Here's the drawing with two shaded views (mm, measured from the low corner). I have some questions. A direction names the side the tool comes from. Give positions to 0.01 mm unless a question says otherwise; leave off trailing zeros. Loops run counter-clockwise (first coordinate to the right, second up) from the corner with the lowest first, then second, coordinate; pieces in that order, holes last. Notation, with made-up numbers: (3.5, 10.5) -> (17.5, 10.5) arc R30 ccw to (17.5, 43.5) -> close; hole circle Ø8 at (5.5, -9.5). An arc over 180 degrees is marked (long way). Answer in a Markdown table with one row per item. Add a question column.
Item 1: If we section it at B-B (y = 17.75): Write out the boundary of the cut face in (x, z), then the cut area to 3 significant figures.
Item 2: If we section it at C-C (y = 13.25): Write out the boundary of the cut face in (x, z).
Item 3: For P1, Ø3, axis at x = 17, z = 13.5, coming from the -Y side; P2, Ø3, axis at x = 19, y = 23.5, coming from the +Z side; P3, Ø2, axis at x = 21.5, z = 16, coming from the +Y side, each with a flat end and sliding along its axis, tell me the tip position at first contact or that it passes through.
Item 4: If we section it at A-A (x = 4.5): Write out the boundary of the cut face in (y, z), then the cut area to 3 significant figures.
Item 5: If I drill on line 1 (Z direction, x = 15.5, y = 24.25); line 2 (Y direction, x = 30, z = 29); line 3 (Y direction, x = 4, z = 16), over which ranges is the centre line in solid material (lowest first)?
Item 6: Which directions (+Z, -Z, +X, -X, +Y, -Y) give clear straight access to the entire face, cutting with the end or side of a thin tool? Please do the marked faces 1 and 2.
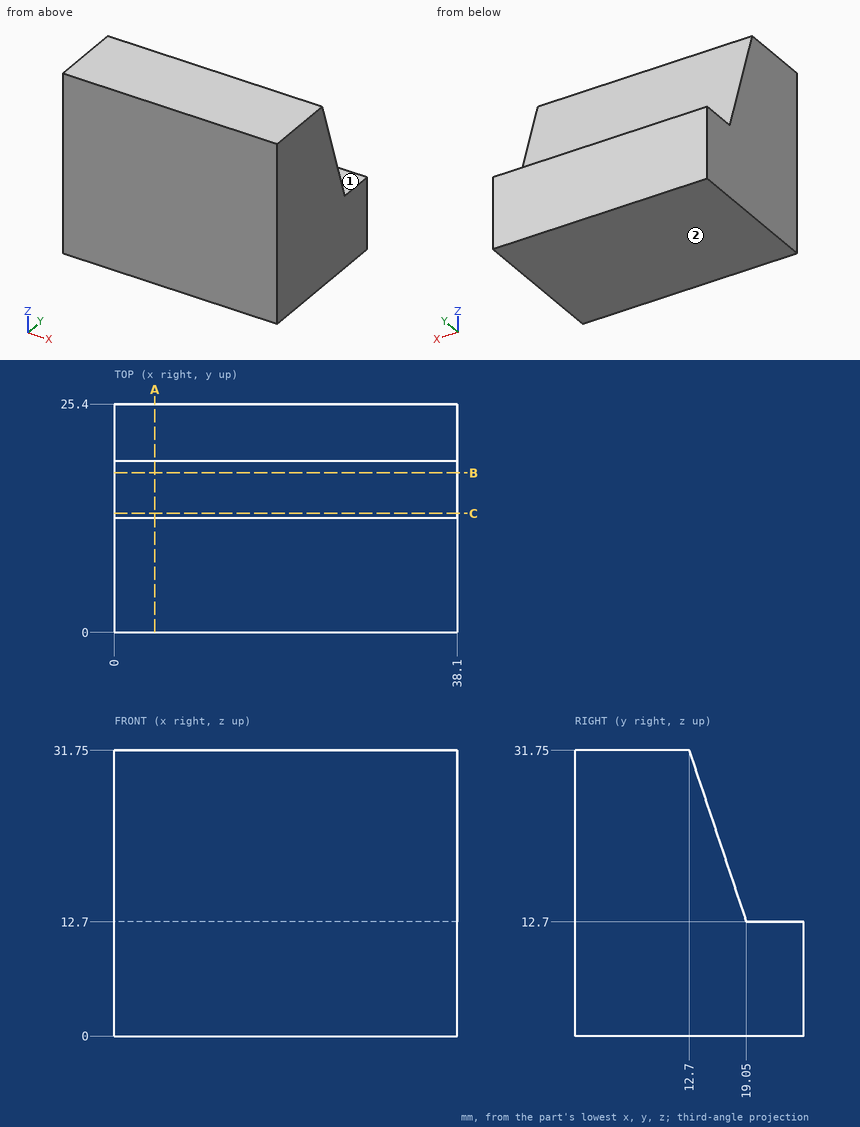
Recorded:
| question | item | result |
|---|---|---|
| 1 | outline | (0, 0) -> (38.1, 0) -> (38.1, 16.6) -> (0, 16.6) -> close |
| 1 | area | 632 mm^2 |
| 2 | outline | (0, 0) -> (38.1, 0) -> (38.1, 30.1) -> (0, 30.1) -> close |
| 3 | P1 | stops at y = 0 |
| 3 | P2 | stops at z = 12.7 |
| 3 | P3 | stops at y = 18.28 |
| 4 | outline | (0, 0) -> (25.4, 0) -> (25.4, 12.7) -> (19.05, 12.7) -> (12.7, 31.75) -> (0, 31.75) -> close |
| 4 | area | 625 mm^2 |
| 5 | line 1 | z = 0 to 12.7 |
| 5 | line 2 | y = 0 to 13.62 |
| 5 | line 3 | y = 0 to 17.95 |
| 6 | face 1 | +Z, +X, -X, +Y |
| 6 | face 2 | -Z, +X, -X, +Y, -Y |
